The listing builds one solid part. Answer for the finished solid, in the listing's coordinates (mm). A direction names the side the tool comes from. Coordinates: 2 decimals unless noted, no trailing zeros. Write each loop counter-clockwise with the first axis right and the second up, starting at its lowest first coordinate (ties: lowest second). Pieces come first, ordered by that corner, then holes.
from build123d import *

# Parameters (mm, degrees)
P_IDAT_VYSUNUT_M1_DEPTH       = 90
ODEBRAT_VYSUNUT_M1_DEPTH      = 87
D_RY_PRO_KOL_K_VELIKOST_MM1_D = 6.5


with BuildPart() as part:
    # Skica1 → Přidat vysunutím1 (new body)
    with BuildSketch(Plane.XY):
        with BuildLine():
            Line((-82.5, 42.5), (82.5, 42.5))
            Line((82.5, 42.5), (82.5, -17.5))
            ThreePointArc((82.5, -17.5), (75.17766953, -35.17766953), (57.5, -42.5))
            Line((57.5, -42.5), (-57.5, -42.5))
            ThreePointArc((-57.5, -42.5), (-75.17766953, -35.17766953), (-82.5, -17.5))
            Line((-82.5, -17.5), (-82.5, 42.5))
        make_face()
    extrude(amount=P_IDAT_VYSUNUT_M1_DEPTH)

    # Skica2 → Odebrat vysunutím1 (cut)
    with BuildSketch(Plane.XY.offset(90)):
        with BuildLine():
            Line((80, -17.5), (80, 40))
            Line((80, 40), (-24, 40))
            Line((-24, 40), (-24, -40))
            Line((-24, -40), (57.5, -40))
            ThreePointArc((57.5, -40), (73.409902577, -33.409902577), (80, -17.5))
        make_face()
        with BuildLine():
            Line((-26, -40), (-26, 40))
            Line((-26, 40), (-80, 40))
            Line((-80, 40), (-80, -17.5))
            ThreePointArc((-80, -17.5), (-73.409902577, -33.409902577), (-57.5, -40))
            Line((-57.5, -40), (-26, -40))
        make_face()
    extrude(amount=-ODEBRAT_VYSUNUT_M1_DEPTH, mode=Mode.SUBTRACT)

    # Díry pro kolík, velikost mm1 (through all)
    with Locations(Plane(origin=(0, 42.5, 0), x_dir=(1, 0, 0), z_dir=(0, 1, 0))):
        with Locations((0, -15), (38, -53), (-38, -53)):
            Hole(D_RY_PRO_KOL_K_VELIKOST_MM1_D / 2)


solid = part.part
Q1. The part is cut by section A-A, the plane x = -38. Write down the section's boundary in (y, z).
Answers below:
outline: (-42.5, 0) - (42.5, 0) - (42.5, 49.75) - (40, 49.75) - (40, 3) - (-40, 3) - (-40, 49.75) - (-42.5, 49.75) - close; (-42.5, 56.25) - (-40, 56.25) - (-40, 90) - (-42.5, 90) - close; (40, 56.25) - (42.5, 56.25) - (42.5, 90) - (40, 90) - close
Q2. The part is cut by section C-C, the plane z = 15. Write down the section's boundary in (x, y), then the cut area to 3 significant figures.
Answers below:
outline: (-82.5, -17.5) arc R25 ccw to (-57.5, -42.5) - (-3.25, -42.5) - (-3.25, -40) - (-24, -40) - (-24, 40) - (-3.25, 40) - (-3.25, 42.5) - (-82.5, 42.5) - close; (3.25, -42.5) - (57.5, -42.5) arc R25 ccw to (82.5, -17.5) - (82.5, 42.5) - (3.25, 42.5) - (3.25, 40) - (80, 40) - (80, -17.5) arc R22.5 cw to (57.5, -40) - (3.25, -40) - close; hole (-80, -17.5) arc R22.5 ccw to (-57.5, -40) - (-26, -40) - (-26, 40) - (-80, 40) - close
area: 1,300 mm2
Q3. The part is cut by section D-D, the plane z = 53. State how many separate pieces and enclosed holes the cut face has, then the cut area to 3 significant figures.
Answers below:
separate pieces: 3
enclosed holes: 0
area: 1,270 mm2
Q4. Find the intervals of material crossed by probe 1 along X at (y, z) = (14, 76.5); probe 2 along X at (y, z) = (40.65, 53); probe 3 along Y at (x, z) = (58.5, 78), in increasing order.
Answers below:
probe 1: x = -82.5 to -80, -26 to -24, 80 to 82.5
probe 2: x = -82.5 to -41.25, -34.75 to 34.75, 41.25 to 82.5
probe 3: y = -42.48 to -39.98, 40 to 42.5
Q5. Given pin 1 (6 mm diameter, centred on x = -41, y = 5, fed in from +Z); pin 2 (4 mm diameter, centred on x = 38, z = 53, fed in from +Y); pin 3 (1 mm diameter, centred on x = -63, z = 65.5, fed in from -Y), each flat-ended and moving along its own axis, determine where each tip first touches the part or whether it passes through.
Answers below:
pin 1: stops at z = 3
pin 2: passes through
pin 3: stops at y = -41.99
Q6. The part is cut by section B-B, the plane z = 35. Write down the section's boundary in (x, y), then the cut area to 3 significant figures.
Answers below:
outline: (-82.5, -17.5) arc R25 ccw to (-57.5, -42.5) - (57.5, -42.5) arc R25 ccw to (82.5, -17.5) - (82.5, 42.5) - (-82.5, 42.5) - close; hole (-80, -17.5) arc R22.5 ccw to (-57.5, -40) - (-26, -40) - (-26, 40) - (-80, 40) - close; hole (-24, -40) - (57.5, -40) arc R22.5 ccw to (80, -17.5) - (80, 40) - (-24, 40) - close
area: 1,330 mm2
Q7. Determine the mould class of faces 3 (the face through (82.5, 13, 44)), 4 (the face through (-74.982, -35.371, 44.37)), 5 (the face through (-41.002, 41.232, 54.245)) for opening direction X: released by +X, released by -X, zero draft, split by the parting line, or undercut.
Answers below:
face 3: released by +X
face 4: released by -X
face 5: undercut
Q8. Which of the six approach directions +Z, -Z, +X, -X, +Y, -Y give full straight-line access (tool end or side, diameter ignored) to faces 1 (the face through (-53, 40, 47)), 2 (the face through (34.998, -41.267, 54.245))?
Answers below:
face 1: +Z
face 2: +Y, -Y
